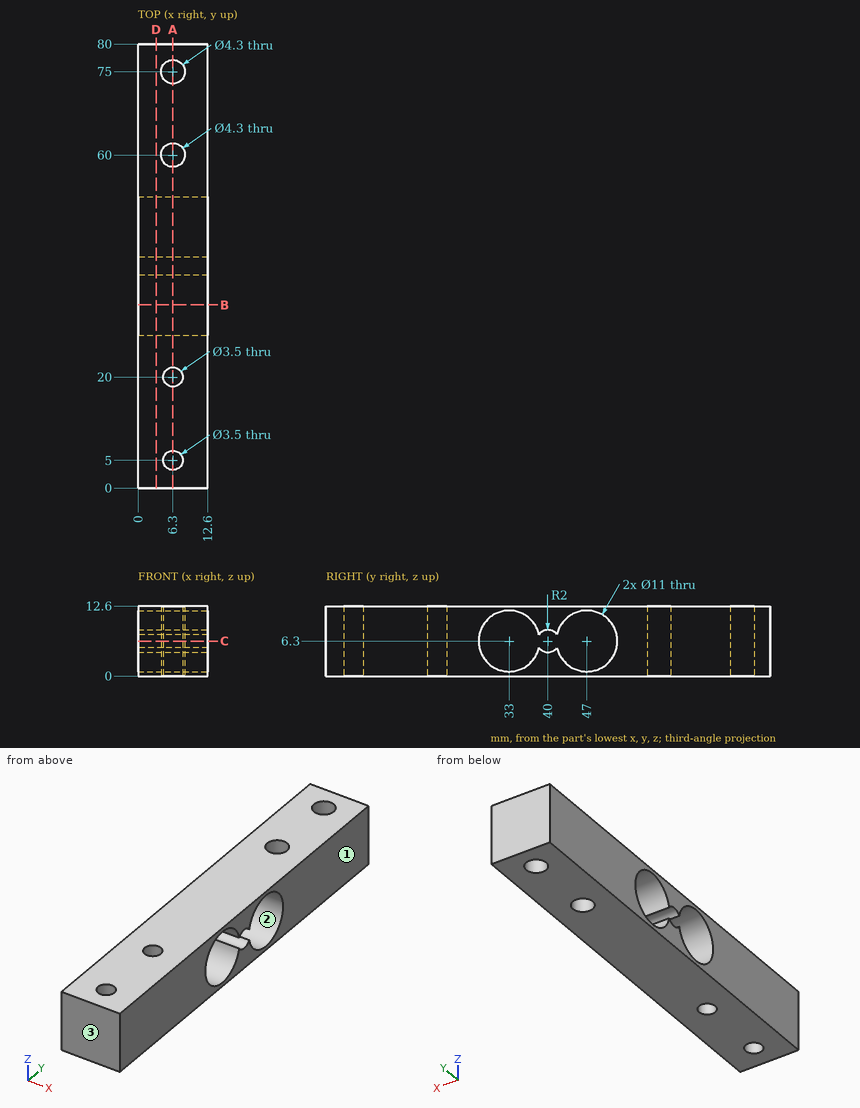
Study the drawing (mm; zero at the part's minimum x, y, z) and answer. Give positions to 0.01 mm unless a question says otherwise; leave off trailing zeros. Write each loop counter-clockwise with the first axis right and the second up, starting at its lowest first coordinate (ties: lowest second). Pieces come first, ordered by that corner, then holes.
(1) The part is cut by section B-B on y = 33. Write down the section's boundary in (x, z), plus the area to 3 significant figures.
Final values:
outline: (0, 0) - (12.6, 0) - (12.6, 0.8) - (0, 0.8) - close; (0, 11.8) - (12.6, 11.8) - (12.6, 12.6) - (0, 12.6) - close
area: 20.2 mm2
(2) The part is cut by section A-A on x = 6.3. Write down the section's boundary in (y, z) (3 decimals).
Final values:
outline: (0, 0) - (3.25, 0) - (3.25, 12.6) - (0, 12.6) - close; (6.75, 0) - (18.25, 0) - (18.25, 12.6) - (6.75, 12.6) - close; (21.75, 0) - (57.85, 0) - (57.85, 12.6) - (21.75, 12.6) - close; (62.15, 0) - (72.85, 0) - (72.85, 12.6) - (62.15, 12.6) - close; (77.15, 0) - (80, 0) - (80, 12.6) - (77.15, 12.6) - close; hole (38.375, 5.134) arc R2 ccw to (41.625, 5.134) arc R5.5 ccw (long way) to (41.625, 7.466) arc R2 ccw to (38.375, 7.466) arc R5.5 ccw (long way) to start
(3) Flat-ended cylindrical pins translate along their axes: pin 1 Ø4 at (x, y) = (6.3, 20) entering from +Z; pin 2 Ø6.5 at (y, z) = (33, 6.3) entering from -X. Find the tip coordinate at first contact, or state that the pin passes through.
Final values:
pin 1: stops at z = 12.6
pin 2: passes through
(4) The part is cut by section C-C on z = 6.3. Write down the section's boundary in (x, y).
Final values:
outline: (0, 0) - (12.6, 0) - (12.6, 27.5) - (0, 27.5) - close; (0, 52.5) - (12.6, 52.5) - (12.6, 80) - (0, 80) - close; hole circle Ø4.3 at (6.3, 60); hole circle Ø4.3 at (6.3, 75); hole circle Ø3.5 at (6.3, 5); hole circle Ø3.5 at (6.3, 20)
(5) The part is cut by section D-D on x = 3.25. Write down the section's boundary in (y, z) (3 decimals).
Final values:
outline: (0, 0) - (80, 0) - (80, 12.6) - (0, 12.6) - close; hole (38.375, 5.134) arc R2 ccw to (41.625, 5.134) arc R5.5 ccw (long way) to (41.625, 7.466) arc R2 ccw to (38.375, 7.466) arc R5.5 ccw (long way) to start
(6) Straight lines are drawn through the part: line 1 (Y direction, x = 6.3, z = 6); line 2 (X direction, y = 5, z = 6); line 3 (Y direction, x = 10.25, z = 7.75). For each, find the intervals that lie inside material, in ascending order.
Final values:
line 1: y = 0 to 3.25, 6.75 to 18.25, 21.75 to 27.51, 52.49 to 57.85, 62.15 to 72.85, 77.15 to 80
line 2: x = 0 to 4.55, 8.05 to 12.6
line 3: y = 0 to 27.69, 38.31 to 38.62, 41.38 to 41.69, 52.31 to 80
(7) The mould has two halves that part along Y. Classify the marked faces 1, 2 and 3: pulls with the +Y half, pulls with the -Y half, needs draft (parallel to the pull), parting line crosses it, or undercut.
Final values:
face 1: needs draft
face 2: undercut
face 3: pulls with the -Y half
